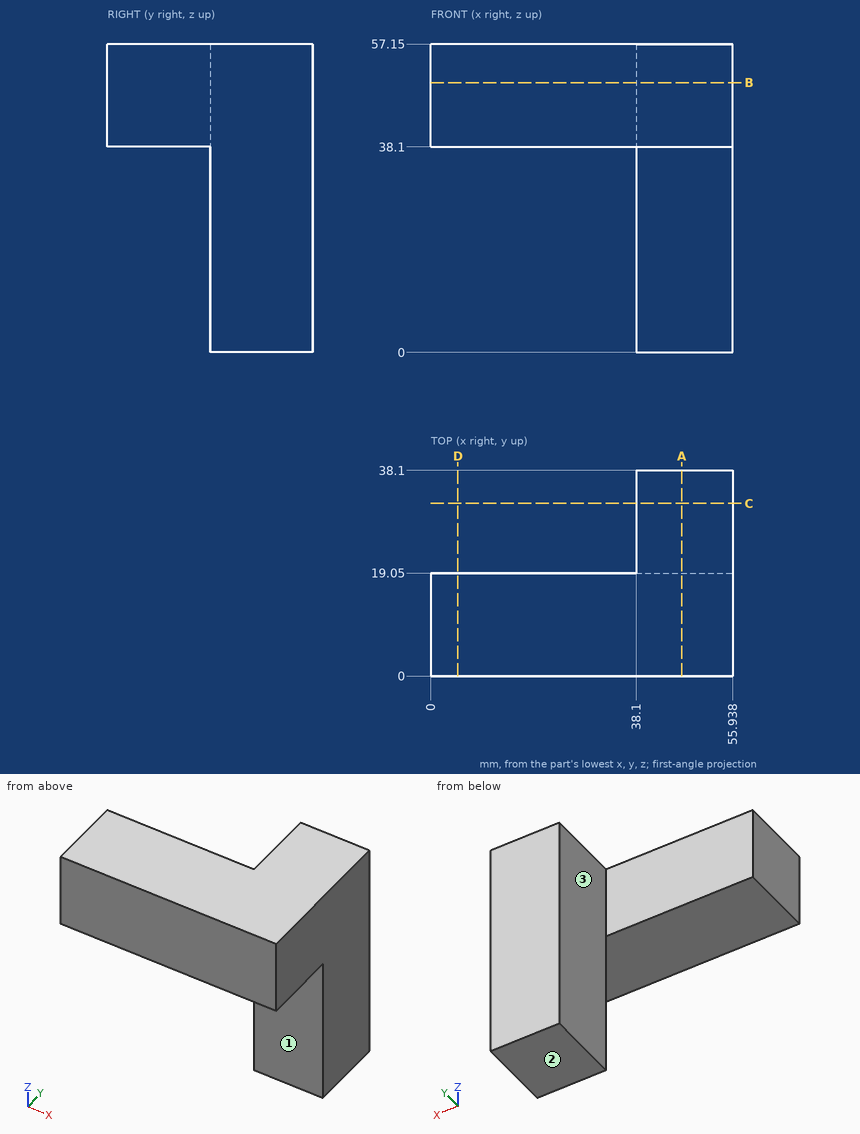
Geometry: see drawing. Coordinates: mm, zero at the bounding-box minimum. A direction names the side the tool comes from. Round coordinates to 2 decimals unless told otherwise and drop trailing zeros. Order: outer loops, then holes, each group sorted by start corner. A loop starts at its lowest first (then second) coordinate and runs counter-clockwise, first axis right, second up. Notation, with made-up numbers: (46, 74) - (56, 74) arc R34 cw to (56, 105) - close; hole circle Ø6 at (-40, 63.5). An arc over 180 degrees is marked (long way). Use a Markdown table: item, result. Add a question column.
1. First-contact query: pin 1 (19.5 mm diameter, centred on x = 45.5, z = 17.5, fed in from -Y); pin 2 (5.5 mm diameter, centred on y = 27.5, z = 39, fed in from -X); pin 3 (10 mm diameter, centred on x = 25, z = 50.5, fed in from +Y). Flat tips, straight axial feed; report the tip coordinate or a pass-through.
2. Line query: probe 1 along Z at (x, y) = (51, 7); probe 2 along X at (y, z) = (23.5, 17.5); probe 3 along Y at (x, z) = (18.5, 39.5). Output: solid intervals per line, ascending.
3. Set-up query: the marked faces 1, 2 and 3. Return all of +Z, -Z, +X, -X, +Y, -Y with unobstructed straight access to the full face (end or side cutting, diameter ignored); none if empty.
4. Section query D-D (x = 5). Return the cut outline in (y, z).
5. Section query C-C (y = 32). Return the cut outline in (x, z).
6. Section query A-A (x = 46.5). Return the cut outline in (y, z), then the cut area to 3 significant figures.
7. Section query B-B (z = 50). Return the cut outline in (x, y), then the cut area to 3 significant figures.
Derived:
| question | item | result |
|---|---|---|
| 1 | pin 1 | y = 19.05 |
| 1 | pin 2 | x = 38.1 |
| 1 | pin 3 | y = 19.05 |
| 2 | probe 1 | 38.1 to 57.15 |
| 2 | probe 2 | 38.1 to 55.94 |
| 2 | probe 3 | 0 to 19.05 |
| 3 | face 1 | -Z, +X, -X, -Y |
| 3 | face 2 | -Z, +X, -X, +Y, -Y |
| 3 | face 3 | +Z, -Z, -X, +Y |
| 4 | outline | (0, 38.1) - (19.05, 38.1) - (19.05, 57.15) - (0, 57.15) - close |
| 5 | outline | (38.1, 0) - (55.94, 0) - (55.94, 57.15) - (38.1, 57.15) - close |
| 6 | outline | (0, 38.1) - (19.05, 38.1) - (19.05, 0) - (38.1, 0) - (38.1, 57.15) - (0, 57.15) - close |
| 6 | area | 1,450 mm2 |
| 7 | outline | (0, 0) - (55.94, 0) - (55.94, 38.1) - (38.1, 38.1) - (38.1, 19.05) - (0, 19.05) - close |
| 7 | area | 1,410 mm2 |
